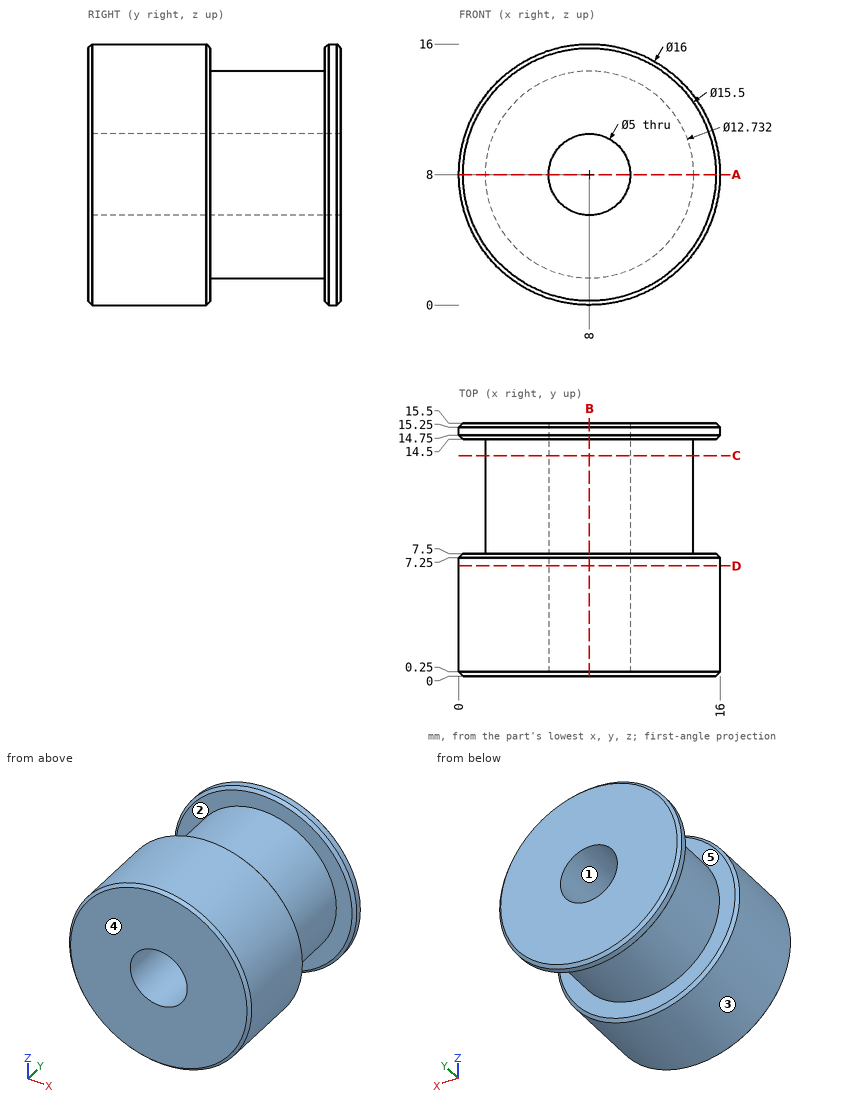
Design review of the part shown in the three views and the two pictorial views. Dimensions are in mm from the part's minimum x, y and z. A direction names the side the tool comes from. Give positions to 0.01 mm unless a question says otherwise; leave off trailing zeros. Write each loop counter-clockwise with the first axis right and the second up, starting at its lowest first coordinate (ties: lowest second). Pieces come first, ordered by that corner, then holes. Notation, with made-up numbers: M 37,11 L 96,11 A34 cw 96,48 Z; hole C 25,47.5 d7. An arc over 180 degrees is marked long. One line per question, with ' | ' between items. Start each with the question number.
Item 1: We need section C-C on y = 13.5. Write out the cut boundary in (x, z), plus the area to 3 significant figures.
Item 2: Wall thickness on line 1 (Y direction, x = 9.5, z = 1.75); line 2 (X direction, y = 8.5, z = 8); line 3 (X direction, y = 5.5, z = 8): over which ranges is each line inside the solid? List them lowest first. Write a range as from..to.
Item 3: For the marked faces 4 and 5, list the 3-axis set-ups (+Z, -Z, +X, -X, +Y, -Y) from which the entire face can be reached by the end or side of a thin tool; tool diameter is ignored.
Item 4: Draft analysis for pull direction X (two halves, no side actions). For the marked faces 1, 2 and 3, state which applies: released by +X, released by -X, zero draft, split by the parting line, or undercut.
Item 5: We need section B-B on x = 8. Write out the cut boundary in (y, z).
Item 6: For pin 1 (2 mm diameter, centred on y = 11, z = 4.5, fed in from -X) (1 decimal); pin 2 (2 mm diameter, centred on y = 4.5, z = 3.5, fed in from +X); pin 3 (6 mm diameter, centred on x = 2.5, y = 13.5, fed in from -Z) (1 decimal), all flat-tipped, find the tip position at first contact; note any pin that passes through.
Item 7: We need section D-D on y = 6.75. Write out the cut boundary in (x, z).
Item 8: We need section A-A on z = 8. Write out the cut boundary in (x, y).
Results found:
1) outline: C 8,8 d12.73; hole C 8,8 d5 | area: 108 mm2
2) line 1: y = 0..7.5, 14.5..15.5 | line 2: x = 1.63..5.5, 10.5..14.37 | line 3: x = 0..5.5, 10.5..16
3) face 4: +Z, -Z, +X, -X, -Y | face 5: none
4) face 1: undercut | face 2: zero draft | face 3: split by the parting line
5) outline: M 0,0.25 L 0.25,0 L 7.25,0 L 7.5,0.25 L 7.5,1.63 L 14.5,1.63 L 14.5,0.25 L 14.75,0 L 15.25,0 L 15.5,0.25 L 15.5,5.5 L 0,5.5 Z; M 0,10.5 L 15.5,10.5 L 15.5,15.75 L 15.25,16 L 14.75,16 L 14.5,15.75 L 14.5,14.37 L 7.5,14.37 L 7.5,15.75 L 7.25,16 L 0.25,16 L 0,15.75 Z
6) pin 1: stops at x = 2.1 | pin 2: stops at x = 15.19 | pin 3: stops at z = 0.5
7) outline: C 8,8 d16; hole C 8,8 d5
8) outline: M 0,0.25 L 0.25,0 L 5.5,0 L 5.5,15.5 L 0.25,15.5 L 0,15.25 L 0,14.75 L 0.25,14.5 L 1.63,14.5 L 1.63,7.5 L 0.25,7.5 L 0,7.25 Z; M 10.5,0 L 15.75,0 L 16,0.25 L 16,7.25 L 15.75,7.5 L 14.37,7.5 L 14.37,14.5 L 15.75,14.5 L 16,14.75 L 16,15.25 L 15.75,15.5 L 10.5,15.5 Z
